Source: CAD feature listing. Evaluate the final solid. Frame: model axes, mm. Round coordinates to 2 decimals unless told otherwise and drop trailing zeros. Order: outer loops, then holes, each group sorted by start corner. A loop starts at its lowest first (then second) coordinate and runs counter-clockwise, first axis right, second up. Notation, with made-up numbers: (21.5, 70) -> (48.5, 70) arc R21 ccw to (48.5, 98) -> close; hole circle Ø2 at (13.25, 74). An arc over 180 degrees is marked (long way). Use a Markdown table: item, result. Add a question column.
```python
from build123d import *

# Parameters (mm, degrees)
F0_W     = 69.230199
F0_H     = 60.010768
F1_DEPTH = 25.4
F2_R     = 6
F3_R     = 7.269466
F4_DEPTH = 25.4


with BuildPart() as f1:
    # F0 (on Front) → F1 (new body)
    with BuildSketch(Plane.XZ):
        with Locations((6.827186, 30.005384)):
            Rectangle(F0_W, F0_H)
    extrude(amount=F1_DEPTH)

    # F2
    f2_edges = [f1.edges().sort_by_distance(p)[0] for p in [
        (41.442286, -12.7, 60.010768),
        (41.442286, -12.7, 0),
        (-27.787913, -12.7, 60.010768),
        (-27.787913, -12.7, 0),
    ]]
    fillet(f2_edges, radius=F2_R)

    # F3 (on face) → F4 (cut, through all)
    with BuildSketch(Plane(origin=(0, 0, 0), x_dir=(-1, 0, 0), z_dir=(0, 1, 0))):
        with Locations((0, 30.005384)):
            Circle(F3_R)
    extrude(amount=-F4_DEPTH, mode=Mode.SUBTRACT)


solid = f1.part
```
1) Line query: probe 1 along Z at (x, y) = (0, -8.5); probe 2 along X at (y, z) = (-13, 34); probe 3 along Z at (x, y) = (-5, -5.75). Output: solid intervals per line, ascending. Write a range as from..to.
2) Section B-B on z = 33. Output: boundary loops of the cut face in (x, y), then the cut area to 3 significant figures.
3) Section A-A on x = 0. Output: boundary loops of the cut face in (y, z), then the cut area to 3 significant figures.
4) Section C-C on y = -22. Output: boundary loops of the cut face in (x, z), then the cut area to 3 significant figures.
5) Draft query along X for faces 1 (the cylindrical face through (0.946, -12.522, 37.213)), 2 (the cylindrical face through (-26.077, -12.878, 58.207)), 3 (the flat face through (6, -13, 60.011)). Return one class per face: pulls with the +X half, pulls with the -X half, needs draft (parallel to the pull), parting line crosses it, or undercut.
Conclusion:
| question | item | result |
|---|---|---|
| 1 | probe 1 | z = 0..22.74, 37.27..60.01 |
| 1 | probe 2 | x = -27.79..-6.07, 6.07..41.44 |
| 1 | probe 3 | z = 0..24.73, 35.28..60.01 |
| 2 | outline | (-27.79, -25.4) -> (-6.62, -25.4) -> (-6.62, 0) -> (-27.79, 0) -> close; (6.62, -25.4) -> (41.44, -25.4) -> (41.44, 0) -> (6.62, 0) -> close |
| 2 | area | 1,420 mm^2 |
| 3 | outline | (-25.4, 0) -> (0, 0) -> (0, 22.74) -> (-25.4, 22.74) -> close; (-25.4, 37.27) -> (0, 37.27) -> (0, 60.01) -> (-25.4, 60.01) -> close |
| 3 | area | 1,150 mm^2 |
| 4 | outline | (-27.79, 6) arc R6 ccw to (-21.79, 0) -> (35.44, 0) arc R6 ccw to (41.44, 6) -> (41.44, 54.01) arc R6 ccw to (35.44, 60.01) -> (-21.79, 60.01) arc R6 ccw to (-27.79, 54.01) -> close; hole circle Ø14.54 at (0, 30.01) |
| 4 | area | 3,960 mm^2 |
| 5 | face 1 | undercut |
| 5 | face 2 | pulls with the -X half |
| 5 | face 3 | needs draft |
